Autodesk Fusion 360 part; units mm, degrees
sketch "Sketch1" plane through (0, 0, 0) normal (0, 1, 0) x (1, 0, 0)
  line L0 (0, -25.4) -> (0, 0)
  line L1 (0, 0) -> (25.4, 0)
  line L2 (12.7, -12.7) -> (11.05, -11.05) construction
  line L3 (3.175, -25.4) -> (3.175, -3.175)
  line L4 (3.175, -3.175) -> (25.4, -3.175)
  line L5 (25.4, -3.175) -> (25.4, 0)
  line L6 (0, -25.4) -> (3.175, -25.4)
  dimension "d1" = 25.4
  dimension "d2" = 25.4
  dimension "d13" = 3.175
extrude "Extrude1" add sketch "Sketch1" along normal blind 139.6
hole "Hole3" at (3.175, 89.6, 14.2875) direction (-1, 0, 0) diameter 6.5 end through all
mirror "Mirror1" about plane through (0, 0, 0) normal (0, 1, 0) of bodies 1 merged
equation "d5 = ( 279.2 / 2 ) * 1 mm"
equation "d27 = ( 22.225 / 2 ) * 1 mm"
Geometry check sheet. Reference: the model listing, model coordinates, mm. A direction names the side the tool comes from. Round coordinates to 2 decimals unless told otherwise and drop trailing zeros. Loops run counter-clockwise (first coordinate to the right, second up) from the corner with the lowest first, then second, coordinate; pieces in that order, holes last. Notation, with made-up numbers: M 46,77.5 L 55,77.5 A29 cw 55,108.5 Z; hole C -20.75,20 d5. An arc over 180 degrees is marked long. Return JSON: item names as keys, results as strings. Group by question number.
(1) Section check A-A, the plane y = -89.6. Enter the section's corners in (x, z) (1 decimal), and give its area (3 significant figures).
(2) Go/stop test with flat-tipped pins: pin 1 (2 mm diameter, centred on x = 14, y = 2, fed in from +Z) (3 decimals); pin 2 (5 mm diameter, centred on y = 89.6, z = 14.29, fed in from +X); pin 3 (2 mm diameter, centred on y = -85.5, z = 18, fed in from +X) (3 decimals). Record where each tip stops, or that it passes through.
(3) Set-up check for faces 5 (the face through (0, -2, 13)), 6 (the face through (3.175, -2, 14)): record each of +Z, -Z, +X, -X, +Y, -Y from which the full face is reachable in a straight line by a thin tool's end or side.
(4) Section check C-C, the plane x = 14.5. Enter the section's corners in (y, z) (3 decimals), and give its area (3 significant figures).
(5) Scan lines: line 1 along Z through (x, y) = (1.3, 89.6); line 2 along X through (y, z) = (51.5, 14.75) (3 decimals). Record each from-to range of solid material in increasing order. Write a range as [from, to].
(6) Mould release check, pull along Y, two halves, no side actions. Record for faces 1 (the face through (1.565, -92.822, 14.711)), 2 (the face through (1.565, 92.773, 14.992)), 3 (the face through (8, -139.6, 2)), 4 (the face through (14, -2, 3.175)): pulls with the +Y half, pulls with the -Y half, needs draft (parallel to the pull), parting line crosses it, or undercut.
(7) Section check D-D, the plane y = 63. Enter the section's corners in (x, z) (3 decimals), and give its area (3 significant figures).
(8) Section check B-B, the plane z = 15. Enter the section's corners in (x, y) (3 decimals), and give its area (3 significant figures).
Data:
{
 "1": {"outline": "M 0,0 L 25.4,0 L 25.4,3.2 L 3.2,3.2 L 3.2,11 L 0,11 Z; M 0,17.5 L 3.2,17.5 L 3.2,25.4 L 0,25.4 Z", "area": "131 mm²"},
 "2": {"pin 1": "z = 3.175", "pin 2": "through", "pin 3": "x = 3.175"},
 "3": {"face 5": "+Z, -Z, -X, +Y, -Y", "face 6": "+Z, +X, +Y, -Y"},
 "4": {"outline": "M -139.6,0 L 139.6,0 L 139.6,3.175 L -139.6,3.175 Z", "area": "886 mm²"},
 "5": {"line 1": "[0, 11.04], [17.54, 25.4]", "line 2": "[0, 3.175]"},
 "6": {"face 1": "undercut", "face 2": "undercut", "face 3": "pulls with the -Y half", "face 4": "needs draft"},
 "7": {"outline": "M 0,0 L 25.4,0 L 25.4,3.175 L 3.175,3.175 L 3.175,25.4 L 0,25.4 Z", "area": "151 mm²"},
 "8": {"outline": "M 0,-139.6 L 3.175,-139.6 L 3.175,-92.771 L 0,-92.771 Z; M 0,-86.429 L 3.175,-86.429 L 3.175,86.429 L 0,86.429 Z; M 0,92.771 L 3.175,92.771 L 3.175,139.6 L 0,139.6 Z", "area": "846 mm²"}
}
